Job drawing, mm, ordinate dimensions from the low corner. One solid piece. A direction names the side the tool comes from. Round coordinates to 2 decimals unless told otherwise and drop trailing zeros. Loops run counter-clockwise (first coordinate to the right, second up) from the corner with the lowest first, then second, coordinate; pieces in that order, holes last. Notation, with made-up numbers: M 50.5,66.25 L 82.5,66.25 A16 ccw 82.5,96.25 Z; hole C 15.5,2.25 d1. An arc over 180 degrees is marked long. Put each result on its own line as item: value. Start each with the question number.
1) Slice it at C-C on y = 16.5. Give the cut face in (x, z) (1 decimal).
2) Slice it at B-B on y = 1.5. Give the cut face in (x, z).
3) Probe line 1 along Y through (x, z) = (2.5, 1.6); line 2 along Z through (x, y) = (2.55, 6); line 3 along X through (y, z) = (12.25, 1.7). List the from-to ranges inside material, lowest first.
4) Drop a flat-ended pin along its axis: pin 1 Ø2 at (x, y) = (3.5, 11.5) entering from -Z. Give the stop position or say it passes through.
5) Which spindle directions (+Z, -Z, +X, -X, +Y, -Y) get a long thin tool onto all of the face, cutting with end or side? Do the marked faces 1 and 2. Say none if no direction does.
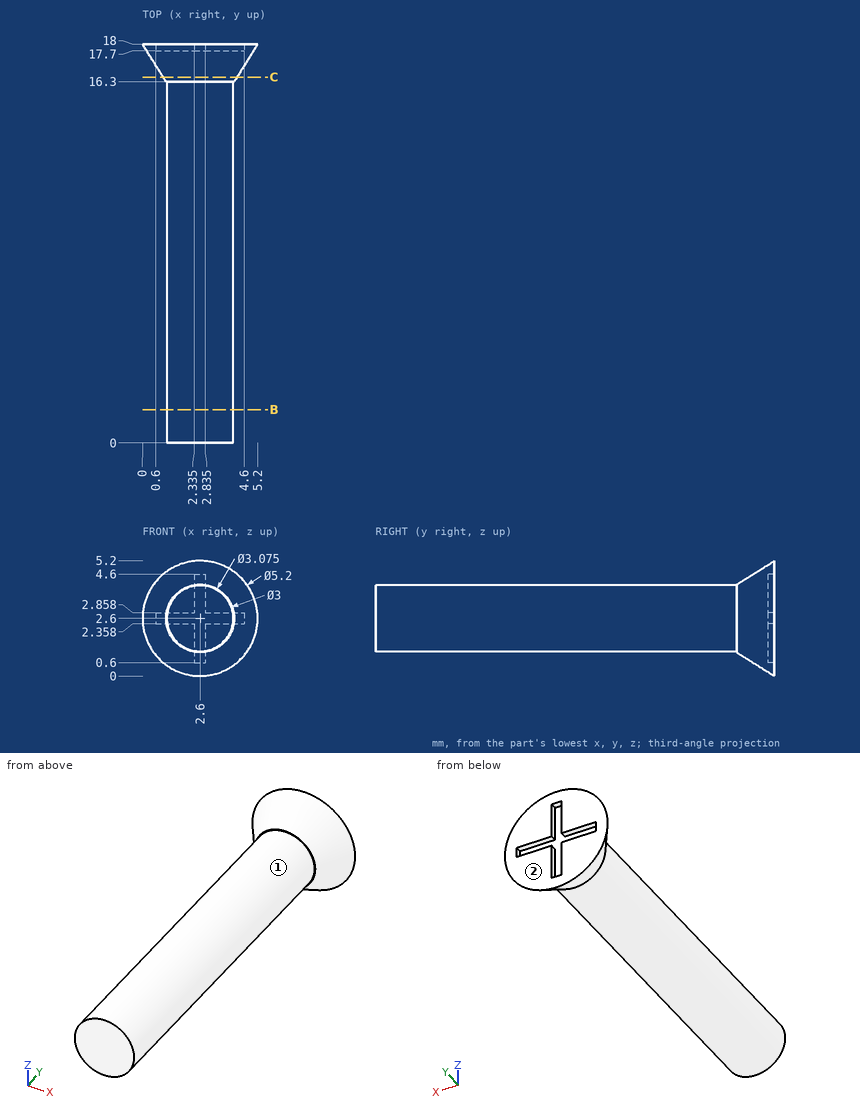
Recorded:
1. outline: C 2.6,2.6 d3.3
2. outline: C 2.6,2.6 d3
3. line 1: y = 0 to 17.7
3. line 2: z = 1.1 to 4.1
3. line 3: x = 1.4 to 3.8
4. pin 1: stops at z = 1.1
5. face 1: -Y
5. face 2: +Z, -Z, +X, -X, +Y
